Verification items for this drawing (mm, ordinates from the low corner). Round coordinates to 2 decimals unless told otherwise and drop trailing zeros. Order: outer loops, then holes, each group sorted by start corner. A loop starts at its lowest first (then second) coordinate and runs counter-clockwise, first axis right, second up. Notation, with made-up numbers: (-3.5, -22) -> (50.5, -22) arc R11 ccw to (50.5, -8) -> close; hole circle Ø8 at (-21.75, 59.5). An arc over 180 degrees is marked (long way). Answer in a Markdown table with one row per item.
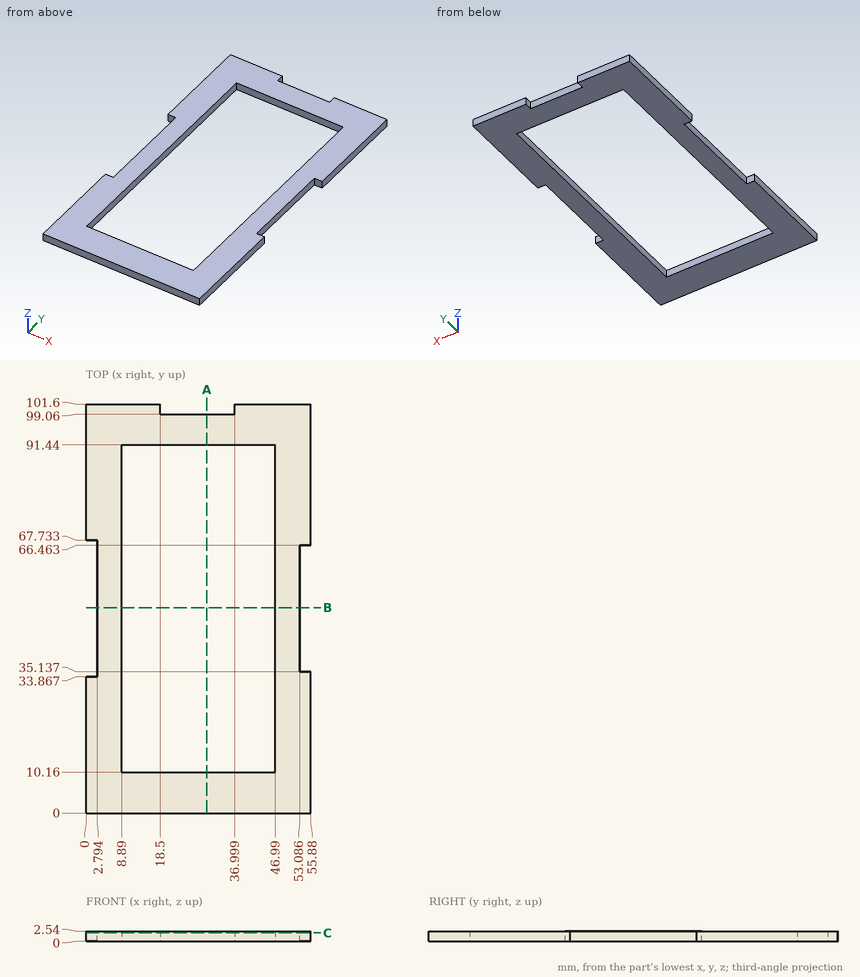
Item 1: Cross-section at B-B (y = 51). Record the boundary of the cut face in (x, z).
Result sheet:
| item | result |
|---|---|
| outline | (2.79, 0) -> (8.89, 0) -> (8.89, 2.54) -> (2.79, 2.54) -> close; (46.99, 0) -> (53.09, 0) -> (53.09, 2.54) -> (46.99, 2.54) -> close |
Item 2: Depth check by flat-ended pin: P1, Ø0.8, axis at x = 27.5, z = 1, coming from the +Y side; P2, Ø0.8, axis at y = 50, z = 1.5, coming from the -X side; P3, Ø0.8, axis at y = 59, z = 1.5, coming from the +X side. Enter the tip coordinate at first touch or a pass-through.
Result sheet:
| item | result |
|---|---|
| P1 | stops at y = 99.06 |
| P2 | stops at x = 2.79 |
| P3 | stops at x = 53.09 |
Item 3: Cross-section at A-A (x = 30). Record the boundary of the cut face in (y, z).
Result sheet:
| item | result |
|---|---|
| outline | (0, 0) -> (10.16, 0) -> (10.16, 2.54) -> (0, 2.54) -> close; (91.44, 0) -> (99.06, 0) -> (99.06, 2.54) -> (91.44, 2.54) -> close |
Item 4: Cross-section at C-C (z = 2.1). Record the boundary of the cut face in (x, y).
Result sheet:
| item | result |
|---|---|
| outline | (0, 0) -> (55.88, 0) -> (55.88, 35.14) -> (53.09, 35.14) -> (53.09, 66.46) -> (55.88, 66.46) -> (55.88, 101.6) -> (37, 101.6) -> (37, 99.06) -> (18.5, 99.06) -> (18.5, 101.6) -> (0, 101.6) -> (0, 67.73) -> (2.79, 67.73) -> (2.79, 33.87) -> (0, 33.87) -> close; hole (8.89, 10.16) -> (46.99, 10.16) -> (46.99, 91.44) -> (8.89, 91.44) -> close |
Item 5: Scan lines: line 1 (Y direction, x = 37.5, z = 1.45); line 2 (X direction, y = 39.5, z = 1.9); line 3 (X direction, y = 71, z = 2.1). Record each from-to range of solid material in increasing order. Write a range as [from, to].
Result sheet:
| item | result |
|---|---|
| line 1 | y = [0, 10.16], [91.44, 101.6] |
| line 2 | x = [2.79, 8.89], [46.99, 53.09] |
| line 3 | x = [0, 8.89], [46.99, 55.88] |
